Part print with two shaded views. Sizes in mm from the minimum x, y, z corner. Round coordinates to 2 decimals unless told otherwise and drop trailing zeros. Order: outer loops, then holes, each group sorted by start corner. A loop starts at its lowest first (then second) coordinate and runs counter-clockwise, first axis right, second up. Notation, with made-up numbers: (4, 73.5) - (29, 73.5) arc R19 ccw to (29, 86.5) - close; hole circle Ø11 at (-23.75, 10). An arc over 180 degrees is marked (long way). Answer as CSV lines item,"result". Start each with the question number.
1. Band-saw the part on A-A on z = 4.5. List the corners of the cut face in (x, y), then the cut area to 3 significant figures.
2. Pull direction X, two halves, no side cores. Call the marked faces 1, 2 and 3: released by +X, released by -X, zero draft, split by the parting line, or undercut.
3. Band-saw the part on C-C on x = 17.5. List the corners of the cut face in (y, z), then the cut area to 3 significant figures.
4. Pin check, flat tip, straight feed: pin 1 Ø6.5 at (x, z) = (17.5, 17.5) entering from +Y. Stop position of the tip, or through.
5. Wall check: line 1 along X through (y, z) = (4, 30.5); line 2 along Z through (x, y) = (17.5, 2). Give the ranges that are in metal, low to high. Write a range as [from, to].
6. Band-saw the part on D-D on z = 17.5. List the corners of the cut face in (x, y), then the cut area to 3 significant figures.
7. Band-saw the part on B-B on y = 2.75. List the corners of the cut face in (x, z), then the cut area to 3 significant figures.
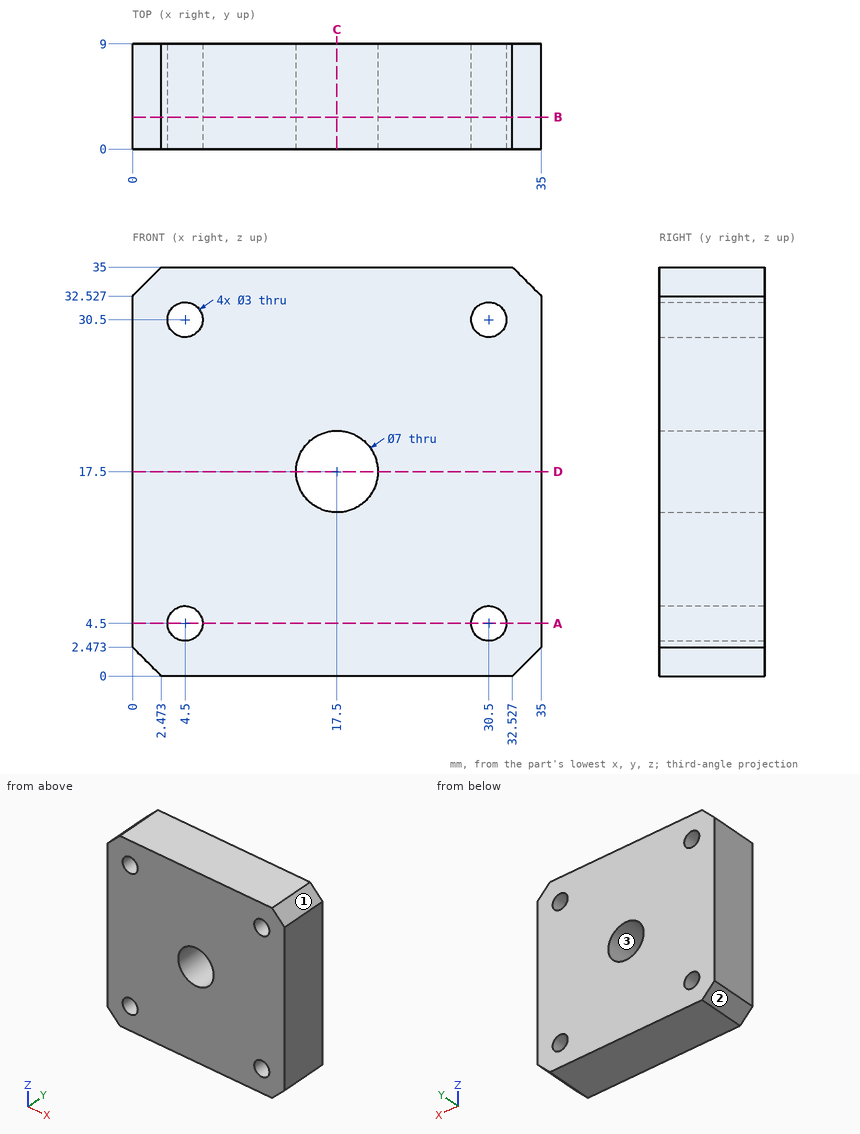
Reply:
1,outline,"(0, 0) - (3, 0) - (3, 9) - (0, 9) - close; (6, 0) - (29, 0) - (29, 9) - (6, 9) - close; (32, 0) - (35, 0) - (35, 9) - (32, 9) - close"
1,area,"261 mm2"
2,face 1,"released by +X"
2,face 2,"released by -X"
2,face 3,"undercut"
3,outline,"(0, 0) - (9, 0) - (9, 14) - (0, 14) - close; (0, 21) - (9, 21) - (9, 35) - (0, 35) - close"
3,area,"252 mm2"
4,pin 1,"passes through"
5,line 1,"x = [0, 3], [6, 29], [32, 35]"
5,line 2,"z = [0, 14], [21, 35]"
6,outline,"(0, 0) - (14, 0) - (14, 9) - (0, 9) - close; (21, 0) - (35, 0) - (35, 9) - (21, 9) - close"
6,area,"252 mm2"
7,outline,"(0, 2.47) - (2.47, 0) - (32.53, 0) - (35, 2.47) - (35, 32.53) - (32.53, 35) - (2.47, 35) - (0, 32.53) - close; hole circle Ø3 at (4.5, 4.5); hole circle Ø3 at (4.5, 30.5); hole circle Ø7 at (17.5, 17.5); hole circle Ø3 at (30.5, 4.5); hole circle Ø3 at (30.5, 30.5)"
7,area,"1,150 mm2"
